```python
from build123d import *

# Parameters (mm, degrees)
SKETCH006_W      = 89
SKETCH006_H      = 84
SKETCH006_R      = 1.524
SKETCH006_W_2    = 5
SKETCH006_H_2    = 7
SKETCH006_W_3    = 64
SKETCH006_H_3    = 41
EXTRUDE006_DEPTH = 3
FILLET008_R      = 1
FILLET009_R      = 1
FILLET010_R      = 1
FILLET012_R      = 1
FILLET013_R      = 1
FILLET014_R      = 1
FILLET015_R      = 1


with BuildPart() as part:
    # Sketch006 → Extrude006 (new body)
    with BuildSketch(Plane.XY):
        with Locations((91.667907, 54.392171)):
            Rectangle(SKETCH006_W, SKETCH006_H)
        with Locations((52.453907, 91.106708)):
            Circle(SKETCH006_R, mode=Mode.SUBTRACT)
        with Locations((130.657907, 91.102171)):
            Circle(SKETCH006_R, mode=Mode.SUBTRACT)
        with Locations((130.707907, 17.767171)):
            Circle(SKETCH006_R, mode=Mode.SUBTRACT)
        with Locations((52.453907, 17.678171)):
            Circle(SKETCH006_R, mode=Mode.SUBTRACT)
        with Locations((91.717396, 28.192171)):
            Rectangle(SKETCH006_W_2, SKETCH006_H_2, mode=Mode.SUBTRACT)
        with Locations((91.667907, 63.392171)):
            Rectangle(SKETCH006_W_3, SKETCH006_H_3, mode=Mode.SUBTRACT)
    extrude(amount=EXTRUDE006_DEPTH)


with BuildPart() as part_1:
    # Extrude006 placement: moved
    add(part.part.moved(Location((0, 0, 30))))

    # Fillet008
    fillet008_edges = [part_1.edges().sort_by_distance(p)[0] for p in [
        (47.167907, 12.392171, 31.5),
    ]]
    fillet(fillet008_edges, radius=FILLET008_R)

    # Fillet009
    fillet009_edges = [part_1.edges().sort_by_distance(p)[0] for p in [
        (59.667907, 42.892171, 31.5),
    ]]
    fillet(fillet009_edges, radius=FILLET009_R)

    # Fillet010
    fillet010_edges = [part_1.edges().sort_by_distance(p)[0] for p in [
        (47.167907, 96.392171, 31.5),
        (47.167907, 54.892171, 33),
    ]]
    fillet(fillet010_edges, radius=FILLET010_R)

    # Fillet012
    fillet012_edges = [part_1.edges().sort_by_distance(p)[0] for p in [
        (129.183907, 17.767171, 33),
    ]]
    fillet(fillet012_edges, radius=FILLET012_R)

    # Fillet013
    fillet013_edges = [part_1.edges().sort_by_distance(p)[0] for p in [
        (132.5248, 17.767171, 32.707107),
        (91.717396, 31.692171, 33),
        (94.217396, 28.192171, 33),
    ]]
    fillet(fillet013_edges, radius=FILLET013_R)

    # Fillet014
    fillet014_edges = [part_1.edges().sort_by_distance(p)[0] for p in [
        (59.667907, 63.892171, 30),
    ]]
    fillet(fillet014_edges, radius=FILLET014_R)

    # Fillet015
    fillet015_edges = [part_1.edges().sort_by_distance(p)[0] for p in [
        (95.217396, 28.692171, 33),
        (94.717396, 24.692171, 33),
        (91.717396, 24.692171, 33),
        (89.217396, 28.192171, 33),
    ]]
    fillet(fillet015_edges, radius=FILLET015_R)


solid = part_1.part
```
Read the model definition and answer for the solid it produces. Units are mm, in the model's axes. A direction names the side the tool comes from. Coordinates: 2 decimals unless noted, no trailing zeros. Loops run counter-clockwise (first coordinate to the right, second up) from the corner with the lowest first, then second, coordinate; pieces in that order, holes last. Notation, with made-up numbers: (30, 76.25) - (78, 76.25) arc R22 cw to (78, 101.25) - close; hole circle Ø8 at (33.25, -38.75). An arc over 180 degrees is marked (long way). Answer in a Markdown table with one row per item.
1. Given pin 1 (2.5 mm diameter, centred on x = 52.45, y = 91.11, fed in from -Z), flat-ended and moving along its own axis, determine where the tip first touches the part or whether it passes through.
Conclusion:
| item | result |
|---|---|
| pin 1 | passes through |
2. Find section A-A, the plane y = 63. Write down the section's boundary in (x, z).
Conclusion:
| item | result |
|---|---|
| outline | (47.17, 30) - (58.67, 30) arc R1 ccw to (59.67, 31) - (59.67, 33) - (48.17, 33) arc R1 ccw to (47.17, 32) - close; (123.67, 30) - (136.17, 30) - (136.17, 33) - (123.67, 33) - close |
3. Straight lines are drawn through the part: line 1 (X direction, y = 64.5, z = 30.85); line 2 (Y direction, x = 108, z = 31.05); line 3 (X direction, y = 27.5, z = 31.4). For each, find the intervals that lie inside material, in ascending order.
Conclusion:
| item | result |
|---|---|
| line 1 | x = 47.17 to 59.66, 123.67 to 136.17 |
| line 2 | y = 12.39 to 42.89, 83.89 to 96.39 |
| line 3 | x = 47.17 to 89.22, 94.22 to 136.17 |
4. Which of the six approach directions +Z, -Z, +X, -X, +Y, -Y give full straight-line access (tool end or side, diameter ignored) to faces 5 (the face through (92, 12.392, 31)), 6 (the face through (94.217, 28, 31))?
Conclusion:
| item | result |
|---|---|
| face 5 | +Z, -Z, +X, -X, -Y |
| face 6 | +Z, -Z |
5. Determine the mould class of faces 1 (the face through (136.168, 54, 31)), 2 (the face through (92, 96.392, 31)), 3 (the face through (50.93, 91.17, 31.48)), 4 (the face through (92, 24.692, 31)) for opening direction X: +X half, -X half, draft (parallel to the pull), parting line (faces both ways), or undercut.
Conclusion:
| item | result |
|---|---|
| face 1 | +X half |
| face 2 | draft |
| face 3 | undercut |
| face 4 | undercut |
6. Find section B-B, the plane x = 91. Write down the section's boundary in (y, z), then the cut area to 3 significant figures.
Conclusion:
| item | result |
|---|---|
| outline | (12.39, 30) - (24.69, 30) - (24.69, 32) arc R1 ccw to (23.69, 33) - (13.39, 33) arc R1 ccw to (12.39, 32) - close; (31.69, 30) - (41.89, 30) arc R1 ccw to (42.89, 31) - (42.89, 33) - (32.69, 33) arc R1 ccw to (31.69, 32) - close; (83.89, 30) - (96.39, 30) - (96.39, 33) - (83.89, 33) - close |
| area | 107 mm² |
